The model under review builds one solid part; all positions refer to its coordinate system, in mm. A direction names the side the tool comes from. Round coordinates to 2 decimals unless told otherwise and drop trailing zeros. Order: outer loops, then holes, each group sorted by start corner. A loop starts at its lowest first (then second) coordinate and runs counter-clockwise, first axis right, second up. Notation, with made-up numbers: M 1,7 L 40,7 A14 ccw 40,29 Z; hole C 76.5,77 d6. An arc over 180 degrees is marked long. Answer as a JSON object with one key per item and string values. Group by question number.
1. To check wall thickness, follow probe 1 along Z at (x, y) = (-35, 0.85); probe 2 along Y at (x, z) = (-27.5, 4); probe 3 along X at (y, z) = (0.25, -15.5). State the ranges of each line that lie inside material, in increasing order. Write a range as [from, to].
2. Clearance check with flat-ended pins moving along their axes: P1, Ø1.3, axis at x = -66.5, z = -10.5, coming from the -Y side; P2, Ø10.5, axis at x = -26.5, z = -9.5, coming from the +Y side. State where each tip first meets the part, or that it passes through.
3. Machinability: for faces 1 (the face through (-21, 0, -5)), 2 (the face through (-60, 0.5, -7)), which of the approach directions +Z, -Z, +X, -X, +Y, -Y give a long, thin tool a straight path to every point of the face, cutting with its end or side? Answer none if there is none.
4. Add section A-A on x = -44. State the section outline as (y, z) points.
5. Add section C-C on z = 8.5. State the section outline as (x, y) points, and give its area (4 significant figures).
6. Add section B-B on y = 0.3. State the section outline as (x, z) points.
```python
from build123d import *

# Parameters (mm, degrees)
SKETCH1_W           = 39.5
SKETCH1_H           = 35
BOSS_EXTRUDE1_DEPTH = 0.5
SKETCH2_W           = 45.379526607
SKETCH2_H           = 1.305742029
SKETCH2_H_2         = 1.314948277
SKETCH2_W_2         = 45.247695687
SKETCH2_H_3         = 1.164010119
SKETCH2_W_3         = 45.478067193
SKETCH2_H_4         = 1.133268544
BOSS_EXTRUDE2_DEPTH = 0.5


with BuildPart() as part:
    # Sketch1 → Boss-Extrude1 (new body)
    with BuildSketch(Plane(origin=(0, 0, 0), x_dir=(1, 0, 0), z_dir=(0, 1, 0))):
        with Locations((-20.235966577, 4.516998197)):
            Rectangle(SKETCH1_W, SKETCH1_H)
    extrude(amount=BOSS_EXTRUDE1_DEPTH)

    # Sketch2 → Boss-Extrude2 (add)
    with BuildSketch(Plane(origin=(0, 0.5, 0), x_dir=(1, 0, 0), z_dir=(0, 1, 0))):
        with Locations((-57.442922572, 3.963636001)):
            Rectangle(SKETCH2_W, SKETCH2_H)
        with Locations((-57.442922572, 7.450727151)):
            Rectangle(SKETCH2_W, SKETCH2_H_2)
        with Locations((-57.377007112, 10.519214372)):
            Rectangle(SKETCH2_W_2, SKETCH2_H_3)
        with Locations((-57.492192865, 13.759786239)):
            Rectangle(SKETCH2_W_3, SKETCH2_H_4)
    extrude(amount=BOSS_EXTRUDE2_DEPTH)


solid = part.part
```
Recorded:
{
 "1": {"probe 1": "z = [-14.33, -13.19], [-11.1, -9.94], [-8.11, -6.79], [-4.62, -3.31]", "probe 2": "y = [0, 0.5]", "probe 3": "x = [-39.99, -0.49]"},
 "2": {"P1": "stops at y = 0.5", "P2": "stops at y = 0.5"},
 "3": {"face 1": "+Z, -Z, +X, -X, -Y", "face 2": "+Z, -Z, -X, -Y"},
 "4": {"outline": "M 0.5,-14.33 L 1,-14.33 L 1,-13.19 L 0.5,-13.19 Z; M 0.5,-11.1 L 1,-11.1 L 1,-9.94 L 0.5,-9.94 Z; M 0.5,-8.11 L 1,-8.11 L 1,-6.79 L 0.5,-6.79 Z; M 0.5,-4.62 L 1,-4.62 L 1,-3.31 L 0.5,-3.31 Z"},
 "5": {"outline": "M -39.99,0 L -0.49,0 L -0.49,0.5 L -39.99,0.5 Z", "area": "19.75 mm²"},
 "6": {"outline": "M -39.99,-22.02 L -0.49,-22.02 L -0.49,12.98 L -39.99,12.98 Z"}
}
